The listing builds one solid part. Answer for the finished solid, in the listing's coordinates (mm). A direction names the side the tool comes from. Give positions to 0.01 mm unless a question says otherwise; leave off trailing zeros. Use one line per item in the form item = value. Start each with the question number.
1. Each of these flat-tipped pins is pushed along its axis until it touches: pin 1 Ø5 at (y, z) = (-8, 6.5) entering from -X; pin 2 Ø4 at (x, z) = (-26.5, 4.5) entering from +Y; pin 3 Ø5 at (x, y) = (3, -14) entering from +Z. Where does it stop, or does it pass through?
2. The mould has two halves that part along Y. Classify faces 1 (the face through (4.06, 7.8, 9.09)), 2 (the face through (-2.313, 1.774, 6.669)), 3 (the face through (-0.5, 15.1, 5)): released by +Y, released by -Y, zero draft, split by the parting line, or undercut.
3. Straight lines are drawn through the part: line 1 (Z direction, x = -6, y = 21); line 2 (X direction, y = 0, z = 2.45); line 3 (Y direction, x = 0, z = 2.3). For each, find the intervals that lie inside material, in ascending order. Write a range as from..to.
4. For faces 4 (the face through (3.345, -0.072, 10.687)), 5 (the face through (0, 0, 2)), determine the directions among +Z, -Z, +X, -X, +Y, -Y from which every point of the face is accessible in a straight line to the end or side of a thin tool.
from build123d import *

# Parameters (mm, degrees)
F2_R = 4.99999


# Not quite as in the source:
# - a fillet or chamfer is up to 0.001 mm smaller than in the source, because OpenCascade refuses the exact size


with BuildPart() as f1:
    # F0 (on Front) → F1 (revolve)
    with BuildSketch(Plane.XZ):
        Polygon((40, 5), (12.8825559993, 5), (7.1957559993, 10.6868), (3.1957559993, 10.6868), (2.6416, 2.762), (2.6416, 2), (0, 2), (0, 0), (40, 0), align=None)
    revolve(axis=Axis((0, 0, -11.1281685531), (0, 0, -1)))

    # F2 (radius 5 in the source; OpenCascade refuses exactly that, so slightly less here)
    f2_edges = [f1.edges().sort_by_distance(p)[0] for p in [
        (-12.882556, 0, 5),
        (-40, 0, 5),
        (-7.195756, 0, 10.6868),
    ]]
    fillet(f2_edges, radius=F2_R)


solid = f1.part
Derived:
q1.pin_1 = -37.19
q1.pin_2 = 29.78
q1.pin_3 = 6.11
q2.face_1 = split by the parting line
q2.face_2 = undercut
q2.face_3 = zero draft
q3.line_1 = 0..5
q3.line_2 = -39.36..-2.64, 2.64..39.36
q3.line_3 = -39.44..-2.64, 2.64..39.44
q4.face_4 = +Z, +X, -X, +Y, -Y
q4.face_5 = +Z
